Autodesk Inventor part; units mm, degrees
ref_plane "YZ Plane" through (0, 0, 0) normal (1, 0, 0) x (0, 1, 0)
ref_plane "XZ Plane" through (0, 0, 0) normal (0, 1, 0) x (-1, 0, 0)
ref_plane "XY Plane" through (0, 0, 0) normal (0, 0, 1) x (1, 0, 0)
sketch "スケッチ2" plane through (0, 0, 0) normal (0, 0, 1) x (1, 0, 0)
  line L0 (0, 0) -> (7, 0) construction
  line L1 (7, 0) -> (7, -27) construction
  line L2 (7, -27) -> (0, -27) construction
  line L3 (0, -27) -> (0, 0) construction
  circle A0 centre (2.5, -3.7) radius 1.6 construction
  circle A1 centre (2.5, -23.3) radius 1.6 construction
  line L4 (5.05, -7.5) -> (0.05, -7.5) construction
  line L5 (0.05, -7.5) -> (0.05, -19.5) construction
  line L6 (0.05, -19.5) -> (5.05, -19.5) construction
  line L7 (5.05, -19.5) -> (5.05, -7.5) construction
  line L8 (0, -7.45) -> (5.1, -7.45) construction
  line L9 (5.1, -7.45) -> (5.1, -19.55) construction
  line L10 (5.1, -19.55) -> (0, -19.55) construction
  line L11 (0, -19.55) -> (0, -7.45) construction
  line L12 (88.7886, 25.8241) -> (57.6759, -5.2886) construction
  line L13 (57.6759, -5.2886) -> (61.2114, -8.8241) construction
  line L14 (61.2114, -8.8241) -> (84.1924, 14.1569) construction
  line L15 (92.3241, 22.2886) -> (88.7886, 25.8241) construction
  line L16 (70.3953, 0.3598) -> (72.1009, 2.0653)
  circle A2 centre (100.1023, -8.117) radius 0.8
  line L17 (7, 0) -> (45.561, -10.3324) construction
  line L18 (7, -27) -> (50.4418, -38.6402) construction
  line L19 (72.4418, -38.6402) -> (106.1477, -10.3575) construction
  line L20 (106.1477, -10.3575) -> (100.2529, -4.1751) construction
  arc A3 (45.561, -10.3324) -> (81.4937, -2.447) centre (55.9138, 28.3046) ccw construction
  line L21 (72.4418, -38.6402) -> (50.4418, -38.6402) construction
  line L22 (39, -8.8) -> (34, -8.8) construction
  line L23 (34, -8.8) -> (34, -33.8) construction
  line L24 (34, -33.8) -> (39, -33.8) construction
  line L25 (39, -33.8) -> (39, -8.8) construction
  circle A4 centre (97.0056, -9.675) radius 0.8 construction
  circle A5 centre (93.6401, -10.5063) radius 0.8 construction
  circle A6 centre (90.1742, -10.5693) radius 0.8
  circle A7 centre (86.7807, -9.8609) radius 0.8 construction
  circle A8 centre (83.6295, -8.4164) radius 0.8 construction
  circle A9 centre (80.8777, -6.3081) radius 0.8
  line L26 (100.2529, -4.1751) -> (104.2516, -8.3688)
  arc A10 (81.4937, -2.447) -> (100.2529, -4.1751) centre (91.6271, 4.8718) ccw construction
  line L27 (39, -15.3) -> (34, -15.3) construction
  line L28 (34, -15.3) -> (34, -27.3) construction
  line L29 (34, -27.3) -> (39, -27.3) construction
  line L30 (39, -27.3) -> (39, -15.3) construction
  line L31 (33.95, -15.25) -> (39.05, -15.25) construction
  line L32 (39.05, -15.25) -> (39.05, -27.35) construction
  line L33 (39.05, -27.35) -> (33.95, -27.35) construction
  line L34 (33.95, -27.35) -> (33.95, -15.25) construction
  circle A11 centre (36.5, -11.5) radius 1.6 construction
  circle A12 centre (36.5, -31.1) radius 1.6 construction
  line L35 (66, -30.5) -> (71, -30.5) construction
  circle A13 centre (68.5, -34.3) radius 1.6 construction
  line L36 (66, -37) -> (71, -37) construction
  line L37 (66, -18.5) -> (66, -30.5) construction
  line L38 (65.95, -30.55) -> (65.95, -18.45) construction
  line L39 (71, -30.5) -> (71, -18.5) construction
  line L40 (66, -12) -> (66, -37) construction
  line L41 (71, -37) -> (71, -12) construction
  line L42 (71.05, -18.45) -> (71.05, -30.55) construction
  line L43 (71.05, -30.55) -> (65.95, -30.55) construction
  circle A14 centre (68.5, -14.7) radius 1.6 construction
  line L44 (71, -18.5) -> (66, -18.5) construction
  line L45 (65.95, -18.45) -> (71.05, -18.45) construction
  line L46 (71, -12) -> (66, -12) construction
  circle A15 centre (71.05, -19.5) radius 1.05 construction
  circle A16 centre (65.95, -19.5) radius 1.05 construction
  circle A17 centre (65.95, -29.5) radius 1.05 construction
  circle A18 centre (71.05, -29.5) radius 1.05 construction
  circle A19 centre (39.05, -16.3) radius 1.05 construction
  circle A20 centre (33.95, -16.3) radius 1.05 construction
  circle A21 centre (33.95, -26.3) radius 1.05 construction
  circle A22 centre (39.05, -26.3) radius 1.05 construction
  circle A23 centre (5.1, -8.5) radius 1.05 construction
  circle A24 centre (0, -8.5) radius 1.05 construction
  circle A25 centre (0, -18.5) radius 1.05 construction
  circle A26 centre (5.1, -18.5) radius 1.05 construction
  line L47 (-3, -7.45) -> (-3, -19.55) construction
  line L48 (-3, -19.55) -> (0, -27) construction
  line L49 (-3, -7.45) -> (0, 0) construction
  circle A27 centre (91.6271, 4.8718) radius 15.5 construction
  arc A28 (77.4664, -6.7113) -> (78.1043, -7.45) centre (91.6271, 4.8718) ccw construction
  line L50 (77.4664, -6.7113) -> (80.2948, -9.5397) construction
  line L51 (104.2516, -8.3688) -> (82.9591, 12.9236) construction
  line L52 (82.9591, 12.9236) -> (84.1924, 14.1569) construction
  line L53 (70.3953, 0.3598) -> (61.2114, -8.8241)
  line L54 (92.3241, 22.2886) -> (95.1525, 19.4602)
  line L55 (95.1525, 19.4602) -> (104.2516, -8.3688)
  line L56 (61.2114, -8.8241) -> (64.0398, -11.6525)
  arc A29 (90.4296, -13.3836) -> (104.2516, -8.3688) centre (91.6271, 4.8718) ccw
  line L57 (64.0398, -11.6525) -> (73.1594, -2.533)
  arc A30 (79.4965, -8.8227) -> (90.4296, -13.3836) centre (91.6271, 4.8718) ccw
  arc A31 (78.1501, -7.5) -> (78.6909, -8.0644) centre (91.6271, 4.8718) ccw construction
  arc A32 (79.4709, -8.8) -> (79.4965, -8.8227) centre (91.6271, 4.8718) ccw
  arc A33 (78.1043, -7.45) -> (78.1501, -7.5) centre (91.6271, 4.8718) ccw construction
  line L58 (84.1924, 14.1569) -> (73.5858, 3.5503) construction
  line L59 (73.5858, 3.5503) -> (71.8887, 5.2473)
  line L60 (71.8887, 5.2473) -> (82.4953, 15.8539)
  line L61 (82.4953, 15.8539) -> (84.1924, 14.1569)
  line L62 (73.5858, 3.5503) -> (82.9591, 12.9236) construction
  line L63 (84.1924, 14.1569) -> (85.6773, 15.6418) construction
  line L64 (84.1924, 14.1569) -> (85.6773, 15.6418) construction
  arc A34 (84.1924, 14.1569) -> (85.6773, 15.6418) centre (84.9349, 14.8993) ccw
  arc A35 (72.1009, 2.0653) -> (73.5858, 3.5503) centre (72.8433, 2.8078) ccw
  arc A36 (85.6773, 15.6418) -> (84.1924, 14.1569) centre (84.9349, 14.8993) ccw construction
  line L65 (85.6773, 15.6418) -> (92.3241, 22.2886) construction
  line L66 (72.1009, 2.0653) -> (73.5858, 3.5503) construction
  arc A37 (73.5858, 3.5503) -> (72.1009, 2.0653) centre (72.8433, 2.8078) ccw construction
  line L67 (85.6773, 15.6418) -> (92.3241, 22.2886)
  line L68 (78.6909, -8.0644) -> (73.1594, -2.533)
  arc A38 (78.6909, -8.0644) -> (79.4709, -8.8) centre (91.6271, 4.8718) ccw
  point P0 (75, 8.5)
  point P1 (91.5446, -20.9171)
  point P2 (82.042, -3.1517)
  point P3 (81.2596, -2.6403)
  point P4 (55.561, -0.3324)
  point P5 (39, -14.2)
  point P6 (34, -14.2)
  point P7 (39, -28.4)
  point P8 (34, -28.4)
  point P9 (79.9568, -9.217)
  dimension "d74" = 7
  dimension "d75" = 27
  dimension "d76" = 3.2
  dimension "d77" = 3.2
  dimension "d78" = 5
  dimension "d79" = 12
  dimension "d80" = 2.5
  dimension "d81" = 2.5
  dimension "d82" = 19.6
  dimension "d83" = 3.7
  dimension "d84" = 7.5
  dimension "d85" = 0.05
  dimension "d86" = 44
  dimension "d87" = 5
  dimension "d88" = 45
  dimension "d89" = 2.5
  dimension "d90" = 22
  dimension "d91" = 75
  dimension "d92" = 8.5
  dimension "d93" = 30
  dimension "d94" = 27
  dimension "d95" = 1.6
  dimension "d96" = 75
  dimension "d97" = 75
  dimension "d98" = 40
  dimension "d99" = 30
  dimension "d100" = 39
  dimension "d101" = 5
  dimension "d102" = 25
  dimension "d103" = 32
  dimension "d104" = 8.8
  dimension "d105" = 77
  dimension "d106" = 22
  dimension "d107" = 12.5
  dimension "d108" = 50
  dimension "d109" = 21
  dimension "d110" = 44
  dimension "d111" = 12
  dimension "d112" = 6.5
  dimension "d113" = 0.05
  dimension "d114" = 3.2
  dimension "d115" = 2.5
  dimension "d116" = 2.7
  dimension "d117" = 3.2
  dimension "d118" = 19.6
  dimension "d119" = 2.5
  dimension "d120" = 5
  dimension "d121" = 25
  dimension "d122" = 12
  dimension "d123" = 6.5
  dimension "d124" = 0.05
  dimension "d125" = 3.2
  dimension "d126" = 2.5
  dimension "d127" = 2.7
  dimension "d128" = 3.2
  dimension "d129" = 19.6
  dimension "d130" = 2.5
  dimension "d131" = 12
  dimension "d132" = 64
  dimension "d133" = 2.1
  dimension "d134" = 2.1
  dimension "d135" = 2.1
  dimension "d136" = 2.1
  dimension "d137" = 2.1
extrude "押し出し2" add sketch "スケッチ2" along normal blind 5
sketch "スケッチ3" plane through (85.6773, 15.6418, 0) normal (-0.7071068, 0.7071068, 0) x (-0.7071068, -0.7071068, 0)
  circle A0 centre (-6.4, 2.5) radius 1.2
  circle A1 centre (31.6, 2.5) radius 1.2
  line L0 (-9.4, 0) -> (0, 0)
  line L1 (-9.4, 0) -> (-9.4, 5)
  line L2 (34.6, 0) -> (34.6, 5)
  line L3 (19.2, 0) -> (34.6, 0)
  point P0 (71.6434, 0)
  dimension "d165" = 2.4
  dimension "d166" = 2.4
  dimension "d167" = 2.5
  dimension "d168" = 3
  dimension "d169" = 3
  dimension "d170" = 2.5
extrude "押し出し3" cut sketch "スケッチ3" against normal through all
fillet "フィレット1" radius 4 2 edges at (104.2516, -8.3688, 2.5) (73.1594, -2.533, 2.5)
sketch "スケッチ5" plane through (0, 0, 5) normal (0, 0, 1) x (1, 0, 0)
  line L0 (89.3543, 19.3187) -> (91.0513, 21.0158) construction
  line L1 (103.3964, -5.7534) -> (95.1525, 19.4602) construction
  line L2 (95.9083, 17.1488) -> (92.4788, 13.7193)
  line L3 (92.4788, 13.7193) -> (99.2403, 6.9578)
  line L4 (90.2028, 20.1673) -> (100.0709, 10.2991) construction
  line L5 (92.3241, 22.2886) -> (85.6773, 15.6418) construction
  line L6 (93.2213, 14.4618) -> (93.9637, 13.7193) construction
  line L7 (93.9637, 13.7193) -> (93.2213, 12.9769) construction
  arc A0 (93.2213, 14.4618) -> (93.2213, 12.9769) centre (93.9637, 13.7193) ccw
  line L8 (93.2213, 14.4618) -> (98.519, 9.1641) construction
  line L9 (95.9083, 17.1488) -> (101.13, 11.927) construction
  line L10 (99.2403, 6.9578) -> (95.9083, 17.1488)
  point P0 (0, 0)
  point P1 (95.9083, 17.1488)
  dimension "d179" = 1.05
  dimension "d180" = 1.9
extrude "押し出し4" cut sketch "スケッチ5" against normal up to surface (5 mm away) contours L10 L3 A0 L2
properties part number "カメラ_メインフレーム" material "アセタール樹脂、黒"
Geometry check sheet. Reference: the model listing, model coordinates, mm. A direction names the side the tool comes from. Round coordinates to 2 decimals unless told otherwise and drop trailing zeros. Loops run counter-clockwise (first coordinate to the right, second up) from the corner with the lowest first, then second, coordinate; pieces in that order, holes last. Notation, with made-up numbers: (-34, -11) - (11, -11) arc R7 ccw to (11, -3) - close; hole circle Ø10 at (-15.75, -1). An arc over 180 degrees is marked (long way). Use a Markdown table: item, result.
Q1. Go/stop test with flat-tipped pins: P1, Ø1.5, axis at x = 93.5, z = 2.5, coming from the +Y side; P2, Ø1.3, axis at x = 100.1, y = -8.12, coming from the +Z side; P3, Ø3, axis at y = 6.5, z = 3, coming from the +X side. Record where each tip stops, or that it passes through.
Solutions:
| item | result |
|---|---|
| P1 | stops at y = 21.86 |
| P2 | passes through |
| P3 | stops at x = 99.88 |
Q2. Cross-section at B-B on x = 98.5. Record the cut outline in (y, z).
Solutions:
| item | result |
|---|---|
| outline | (-12.08, 0) - (7.7, 0) - (7.7, 5) - (-12.08, 5) - close |
Q3. Material ranges on line 1 (X direction, y = -8.5, z = 3.05); line 2 (X direction, y = 14.5, z = 4.1); line 3 (Y direction, x = 81, z = 1), recorded low to high.
Solutions:
| item | result |
|---|---|
| line 1 | x = 61.54 to 63.62, 66.64 to 67.19, 79.14 to 99.4, 100.8 to 103.3 |
| line 2 | x = 81.14 to 83.85, 85.91 to 93.26 |
| line 3 | y = -10.02 to -7.1, -5.52 to 14.36 |
Q4. Draft check along Y on faces 4 (the cylindrical face through (81.617, -6.002, 2.465)), 5 (the flat face through (83.33, 15.02, 2.46)), 6 (the cylindrical face through (92.914, 13.731, 2.535)), 7 (the cylindrical face through (73.2, -4.19, 2.54)). Enter one of: released by +Y, released by -Y, zero draft, split by the parting line, or undercut.
Solutions:
| item | result |
|---|---|
| face 4 | undercut |
| face 5 | released by +Y |
| face 6 | undercut |
| face 7 | released by -Y |
Q5. Cross-section at A-A on y = 11. Record the cut outline in (x, z), plus the area to 3 significant figures.
Solutions:
| item | result |
|---|---|
| outline | (77.64, 0) - (95.2, 0) - (95.2, 5) - (77.64, 5) - close |
| area | 87.8 mm2 |
Q6. Access from +Z, -Z, +X, -X, +Y, -Y to the whole of each face (thin tool, end or side, straight path). Record for faces 1 (the cylindrical face through (85.69, 14.17, 2.46)), 2 (the flat face through (67.14, -8.55, 2.46)), 3 (the flat face through (96.2, 10, 2.5)).
Solutions:
| item | result |
|---|---|
| face 1 | +Z, -Z |
| face 2 | +Z, -Z, -Y |
| face 3 | +Z, -Z, +X |
